Read the model definition and answer for the solid it produces. Units are mm, in the model's axes. Face numbers are marked on the shaded views. A direction names the side the tool comes from. Coordinates: 2 decimals unless noted, no trailing zeros. Loops run counter-clockwise (first coordinate to the right, second up) from the corner with the lowest first, then second, coordinate; pieces in that order, holes last. Notation, with made-up numbers: (-22.5, 20.25) - (27.5, 20.25) arc R30 ccw to (27.5, 42.25) - close; hole circle Ø1 at (13.25, -29). An arc over 180 degrees is marked (long way). One line per item, written item: value. Start each with the question number.
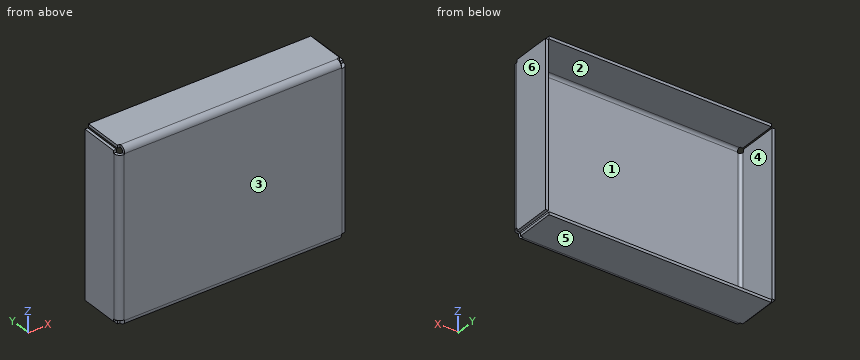
from build123d import *

# Parameters (mm, degrees)
SKETCH1_W              = 400
SKETCH1_H              = 300
BOSS_EXTRUDE1_DEPTH    = 80
SHELL1_T               = -5
CONVERT_SOLID1_START   = -200
CONVERT_SOLID1_DEPTH   = 400
CONVERT_SOLID1_2_DEPTH = 6.414213562
CONVERT_SOLID1_START_2 = 193.585786438
CONVERT_SOLID1_3_DEPTH = 6.414213562
CONVERT_SOLID1_START_3 = -193.585786438
CONVERT_SOLID1_4_DEPTH = 4.835786438
CONVERT_SOLID1_START_4 = 188.75
CONVERT_SOLID1_5_DEPTH = 4.835786438
CONVERT_SOLID1_START_5 = -188.75
CONVERT_SOLID1_6_DEPTH = 377.5
CONVERT_SOLID1_START_6 = -138.75
CONVERT_SOLID1_7_DEPTH = 277.5
CONVERT_SOLID1_8_DEPTH = 277.5


with BuildPart() as part:
    # Sketch1 → Boss-Extrude1 (new body)
    with BuildSketch(Plane(origin=(0, 0, 0), x_dir=(1, 0, 0), z_dir=(0, 1, 0))):
        Rectangle(SKETCH1_W, SKETCH1_H)
    extrude(amount=BOSS_EXTRUDE1_DEPTH)

    # Shell1
    shell1_openings = [part.faces().sort_by_distance(p)[0] for p in [
        (0, 80, 0),
    ]]
    offset(amount=SHELL1_T, openings=shell1_openings, kind=Kind.INTERSECTION)

    # Convert-Solid1: read off the stored shape, not the designer's step
    # Convert-Solid1 outline → Convert-Solid1 (cut)
    with BuildSketch(Plane.YZ.offset(CONVERT_SOLID1_START)):
        with BuildLine():
            Line((11.25, -138.75), (5, -138.75))
            Line((5, -138.75), (5, -140))
            ThreePointArc((5, -140), (6.464466094, -143.535533906), (10, -145))
            Line((10, -145), (80, -145))
            Line((80, -145), (80, -143.585786438))
            Line((80, -143.585786438), (11.25, -143.585786438))
            Line((11.25, -143.585786438), (11.25, -138.75))
        make_face()
        with BuildLine():
            Line((5, 140), (5, 138.75))
            Line((5, 138.75), (11.25, 138.75))
            Line((11.25, 138.75), (11.25, 143.585786438))
            Line((11.25, 143.585786438), (80, 143.585786438))
            Line((80, 143.585786438), (80, 145))
            Line((80, 145), (10, 145))
            ThreePointArc((10, 145), (6.464466094, 143.535533906), (5, 140))
        make_face()
        with BuildLine():
            ThreePointArc((10, -150), (2.928932188, -147.071067812), (0, -140))
            Line((0, -140), (0, -150))
            Line((0, -150), (10, -150))
        make_face()
        with BuildLine():
            Line((0, 150), (0, 140))
            ThreePointArc((0, 140), (2.928932188, 147.071067812), (10, 150))
            Line((10, 150), (0, 150))
        make_face()
    extrude(amount=CONVERT_SOLID1_DEPTH, mode=Mode.SUBTRACT)

    # Convert-Solid1 2 outline → Convert-Solid1 2 (cut)
    with BuildSketch(Plane.YZ.offset(CONVERT_SOLID1_START)):
        with BuildLine():
            Line((5, -140), (5, -138.75))
            Line((5, -138.75), (0, -138.75))
            Line((0, -138.75), (0, -140))
            ThreePointArc((0, -140), (2.928932188, -147.071067812), (10, -150))
            Line((10, -150), (80, -150))
            Line((80, -150), (80, -145))
            Line((80, -145), (10, -145))
            ThreePointArc((10, -145), (6.464466094, -143.535533906), (5, -140))
        make_face()
        with BuildLine():
            Line((0, 138.75), (5, 138.75))
            Line((5, 138.75), (5, 140))
            ThreePointArc((5, 140), (6.464466094, 143.535533906), (10, 145))
            Line((10, 145), (80, 145))
            Line((80, 145), (80, 150))
            Line((80, 150), (10, 150))
            ThreePointArc((10, 150), (2.928932188, 147.071067812), (0, 140))
            Line((0, 140), (0, 138.75))
        make_face()
    extrude(amount=CONVERT_SOLID1_2_DEPTH, mode=Mode.SUBTRACT)

    # Convert-Solid1 3 outline → Convert-Solid1 3 (cut)
    with BuildSketch(Plane.YZ.offset(CONVERT_SOLID1_START_2)):
        with BuildLine():
            Line((5, -140), (5, -138.75))
            Line((5, -138.75), (0, -138.75))
            Line((0, -138.75), (0, -140))
            ThreePointArc((0, -140), (2.928932188, -147.071067812), (10, -150))
            Line((10, -150), (80, -150))
            Line((80, -150), (80, -145))
            Line((80, -145), (10, -145))
            ThreePointArc((10, -145), (6.464466094, -143.535533906), (5, -140))
        make_face()
        with BuildLine():
            Line((0, 138.75), (5, 138.75))
            Line((5, 138.75), (5, 140))
            ThreePointArc((5, 140), (6.464466094, 143.535533906), (10, 145))
            Line((10, 145), (80, 145))
            Line((80, 145), (80, 150))
            Line((80, 150), (10, 150))
            ThreePointArc((10, 150), (2.928932188, 147.071067812), (0, 140))
            Line((0, 140), (0, 138.75))
        make_face()
    extrude(amount=CONVERT_SOLID1_3_DEPTH, mode=Mode.SUBTRACT)

    # Convert-Solid1 4 outline → Convert-Solid1 4 (cut)
    with BuildSketch(Plane.YZ.offset(CONVERT_SOLID1_START_3)):
        with BuildLine():
            Line((5, -145), (5, -138.75))
            Line((5, -138.75), (0, -138.75))
            Line((0, -138.75), (0, -140))
            ThreePointArc((0, -140), (2.928932188, -147.071067812), (10, -150))
            Line((10, -150), (11.25, -150))
            Line((11.25, -150), (11.25, -145))
            Line((11.25, -145), (5, -145))
        make_face()
        with BuildLine():
            Line((0, 138.75), (5, 138.75))
            Line((5, 138.75), (5, 145))
            Line((5, 145), (11.25, 145))
            Line((11.25, 145), (11.25, 150))
            Line((11.25, 150), (10, 150))
            ThreePointArc((10, 150), (2.928932188, 147.071067812), (0, 140))
            Line((0, 140), (0, 138.75))
        make_face()
    extrude(amount=CONVERT_SOLID1_4_DEPTH, mode=Mode.SUBTRACT)

    # Convert-Solid1 5 outline → Convert-Solid1 5 (cut)
    with BuildSketch(Plane.YZ.offset(CONVERT_SOLID1_START_4)):
        with BuildLine():
            Line((5, -145), (5, -138.75))
            Line((5, -138.75), (0, -138.75))
            Line((0, -138.75), (0, -140))
            ThreePointArc((0, -140), (2.928932188, -147.071067812), (10, -150))
            Line((10, -150), (11.25, -150))
            Line((11.25, -150), (11.25, -145))
            Line((11.25, -145), (5, -145))
        make_face()
        with BuildLine():
            Line((0, 138.75), (5, 138.75))
            Line((5, 138.75), (5, 145))
            Line((5, 145), (11.25, 145))
            Line((11.25, 145), (11.25, 150))
            Line((11.25, 150), (10, 150))
            ThreePointArc((10, 150), (2.928932188, 147.071067812), (0, 140))
            Line((0, 140), (0, 138.75))
        make_face()
    extrude(amount=CONVERT_SOLID1_5_DEPTH, mode=Mode.SUBTRACT)

    # Convert-Solid1 6 outline → Convert-Solid1 6 (add)
    with BuildSketch(Plane.YZ.offset(CONVERT_SOLID1_START_5)):
        with BuildLine():
            ThreePointArc((10, -145), (6.464466094, -143.535533906), (5, -140))
            Line((5, -140), (5, -145))
            Line((5, -145), (10, -145))
        make_face()
        with BuildLine():
            Line((5, 145), (5, 140))
            ThreePointArc((5, 140), (6.464466094, 143.535533906), (10, 145))
            Line((10, 145), (5, 145))
        make_face()
    extrude(amount=CONVERT_SOLID1_6_DEPTH)

    # Convert-Solid1 7 outline → Convert-Solid1 7 (cut)
    with BuildSketch(Plane.XY.offset(CONVERT_SOLID1_START_6)):
        with BuildLine():
            ThreePointArc((200, 10), (197.071067812, 2.928932188), (190, 0))
            Line((190, 0), (200, 0))
            Line((200, 0), (200, 10))
        make_face()
        with BuildLine():
            ThreePointArc((-190, 0), (-197.071067812, 2.928932188), (-200, 10))
            Line((-200, 10), (-200, 0))
            Line((-200, 0), (-190, 0))
        make_face()
    extrude(amount=CONVERT_SOLID1_7_DEPTH, mode=Mode.SUBTRACT)

    # Convert-Solid1 8 outline → Convert-Solid1 8 (add)
    with BuildSketch(Plane.XY.offset(CONVERT_SOLID1_START_6)):
        with BuildLine():
            ThreePointArc((195, 10), (193.535533906, 6.464466094), (190, 5))
            Line((190, 5), (195, 5))
            Line((195, 5), (195, 10))
        make_face()
        with BuildLine():
            ThreePointArc((-190, 5), (-193.535533906, 6.464466094), (-195, 10))
            Line((-195, 10), (-195, 5))
            Line((-195, 5), (-190, 5))
        make_face()
    extrude(amount=CONVERT_SOLID1_8_DEPTH)


solid = part.part
1) Determine the mould class of the marked faces 4, 5 and 6 for opening direction X: released by +X, released by -X, zero draft, split by the parting line, or undercut.
2) Section B-B, the plane z = 85.5 is taken. Determine the outline of the cut face in (x, y), and give its area (3 significant figures).
3) Straight lines are drawn through the part: L1, parallel to Z at x = -159, y = 49; L2, parallel to X at y = 28, z = 137; L3, parallel to Y at x = 0, z = 34.5. For each, find the intervals that lie inside material, in ascending order.
4) For the marked faces 1, 2 and 3, determine the directions among +Z, -Z, +X, -X, +Y, -Y from which every point of the face is accessible in a straight line to the end or side of a thin tool.
5) Section A-A, the plane y = 19 is taken. Determine the outline of the cut face in (x, z).
6) Flat-ended cylindrical pins translate along their axes: P1, Ø1.5, axis at y = 31, z = 147.5, coming from the +X side; P2, Ø1.5, axis at x = -198.5, y = 39, coming from the -Z side; P3, Ø5.5, axis at x = -198, z = -140.5, coming from the -Y side; P4, Ø2, axis at x = 44, z = 29.5, coming from the -Y side. Find the tip coordinate at first contact, or state that the pin passes through.
7) Section C-C, the plane x = 49 is taken. Determine the outline of the cut face in (y, z).
Answer below:
1. face 4: undercut
1. face 5: zero draft
1. face 6: released by +X
2. outline: (-200, 10) arc R10 ccw to (-190, 0) - (190, 0) arc R10 ccw to (200, 10) - (200, 80) - (195, 80) - (195, 10) arc R5 cw to (190, 5) - (-190, 5) arc R5 cw to (-195, 10) - (-195, 80) - (-200, 80) - close
2. area: 2,720 mm2
3. L1: -150 to -145, 145 to 150
3. L2: -200 to -195, 195 to 200
3. L3: 0 to 5
4. face 1: +Y
4. face 2: +X, -X, +Y
4. face 3: +Z, -Z, +X, -X, -Y
5. outline: (-200, -143.59) - (-195, -143.59) - (-195, 143.59) - (-200, 143.59) - close; (-193.59, -150) - (193.59, -150) - (193.59, -145) - (-193.59, -145) - close; (-193.59, 145) - (193.59, 145) - (193.59, 150) - (-193.59, 150) - close; (195, -143.59) - (200, -143.59) - (200, 143.59) - (195, 143.59) - close
6. P1: x = 193.59
6. P2: z = -143.59
6. P3: y = 1.91
6. P4: y = 0
7. outline: (0, -140) arc R10 ccw to (10, -150) - (80, -150) - (80, -145) - (10, -145) arc R5 cw to (5, -140) - (5, 140) arc R5 cw to (10, 145) - (80, 145) - (80, 150) - (10, 150) arc R10 ccw to (0, 140) - close
